Solid Edge part; units mm, degrees
sketch "Sketch1" plane through (0, 0, 0) normal (0, -1, 0) x (1, 0, 0)
  line L0 (0, 0) -> (0, 290)
  line L1 (0, 290) -> (16, 290)
  line L2 (16, 290) -> (16, 250)
  line L3 (16, 250) -> (10, 250)
  line L4 (10, 250) -> (10, 40)
  line L5 (10, 40) -> (6, 40)
  line L6 (6, 40) -> (6, 22)
  line L7 (6, 22) -> (5, 22)
  line L8 (5, 22) -> (5, 0)
  line L9 (5, 0) -> (0, 0)
  dimension "D1" = 10
  dimension "D2" = 16
  dimension "D3" = 5
  dimension "D4" = 6
revolve "RevolvedProtrusion1" add sketch "Sketch1" angle 360 about axis through (0, 0, 54) along (0, 0, -1)
sketch "Sketch2" plane through (0, 0, 0) normal (1, 0, 0) x (0, 1, 0)
  circle A0 centre (0, 270) radius 5
extrude "Cutout1" cut sketch "Sketch2" along normal mid plane 303.6008
sketch "Sketch3" plane through (0, 0, 0) normal (0, -1, 0) x (1, 0, 0)
  circle A0 centre (0, 270) radius 5
extrude "ExtrudedCutout_2" cut sketch "Sketch3" along normal mid plane 286.0793
fillet "Round_1" radius 3 1 edges at (-16, 0, 290)
cosmetic_thread "Thread_1" thread depth 170
cosmetic_thread "Thread1"
chamfer "Chamfer_1" distance 1 angle 45 1 edges at (-10, 0, 40)
chamfer "Chamfer_2" distance 1 angle 45 1 edges at (-5, 0, 0)
properties material "Fe 410 W"
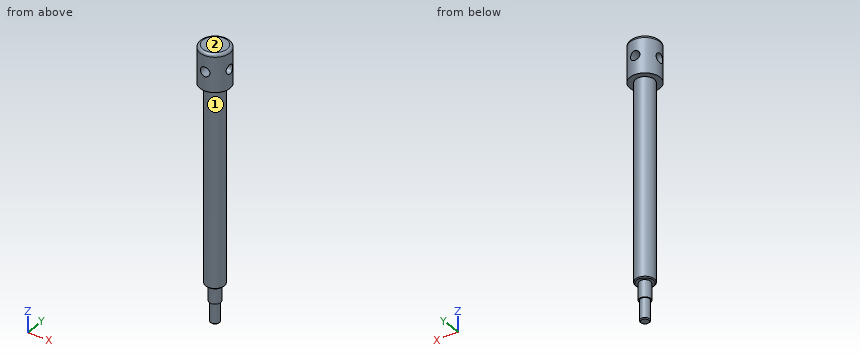
Read the model definition and answer for the solid it produces. Units are mm, in the model's axes. Face numbers are marked on the shaded views. A direction names the side the tool comes from. Coordinates: 2 decimals unless noted, no trailing zeros. Loops run counter-clockwise (first coordinate to the right, second up) from the corner with the lowest first, then second, coordinate; pieces in that order, holes last. Notation, with made-up numbers: (30.5, 34.5) - (55.5, 34.5) arc R22 ccw to (55.5, 63.5) - close; hole circle Ø7 at (89, 46). An arc over 180 degrees is marked (long way). Answer in a Markdown table with one row per item.
Q1. Straight lines are drawn through the part: line 1 along Z through (x, y) = (5.5, 0); line 2 along Z through (x, y) = (-11.75, 0); line 3 along X through (y, z) = (8, 233.5). For each, find the intervals that lie inside material, in ascending order. Write a range as [from, to].
Here are the results:
| item | result |
|---|---|
| line 1 | z = [22, 265], [275, 290] |
| line 2 | z = [250, 265], [275, 290] |
| line 3 | x = [-6, 6] |
Q2. Find section A-A on z = 270. Write down the section's boundary in (x, y).
Here are the results:
| item | result |
|---|---|
| outline | (-15.2, -5) arc R16 ccw to (-5, -15.2) - (-5, -5) - close; (-15.2, 5) - (-5, 5) - (-5, 15.2) arc R16 ccw to start; (5, -15.2) arc R16 ccw to (15.2, -5) - (5, -5) - close; (5, 5) - (15.2, 5) arc R16 ccw to (5, 15.2) - close |
Q3. Find section B-B on z = 43.5. Write down the section's boundary in (x, y).
Here are the results:
| item | result |
|---|---|
| outline | circle Ø20 at (0, 0) |
Q4. For the marked faces 1 and 2, determine the directions among +Z, -Z, +X, -X, +Y, -Y from which every point of the face is accessible in a straight line to the end or side of a thin tool.
Here are the results:
| item | result |
|---|---|
| face 1 | -Z |
| face 2 | +Z, +X, -X, +Y, -Y |
Q5. Given P1, Ø6, axis at x = 3, z = 212, coming from the +Y side; P2, Ø10, axis at y = -2.5, z = 171, coming from the -X side; P3, Ø8, axis at y = 3, z = 206.5, coming from the +X side; P4, Ø1.5, axis at y = 12.5, z = 238, coming from the +X side, each flat-ended and moving along its own axis, determine where each tip first touches the part or whether it passes through.
Here are the results:
| item | result |
|---|---|
| P1 | stops at y = 10 |
| P2 | stops at x = -10 |
| P3 | stops at x = 10 |
| P4 | passes through |
